Autodesk Inventor part; units mm, degrees
ref_plane "YZ Plane" through (0, 0, 0) normal (1, 0, 0) x (0, 1, 0)
ref_plane "XZ Plane" through (0, 0, 0) normal (0, 1, 0) x (-1, 0, 0)
ref_plane "XY Plane" through (0, 0, 0) normal (0, 0, 1) x (1, 0, 0)
sketch "Sketch1" plane through (0, 0, 0) normal (0, 1, 0) x (-1, 0, 0)
  circle A0 centre (0, 0) radius 3.75
  dimension "d0" = 7.5
extrude "Extrusion1" add sketch "Sketch1" along normal blind 18.4
sketch "Sketch2" plane through (0, 0, 0) normal (1, 0, 0) x (0, 1, 0)
  circle A0 centre (3.75, 0) radius 3.75
  line L0 (0, -3.75) -> (0, 3.75)
  point P0 (0, 0)
  dimension "d3" = 7.5
extrude "Extrusion2" add sketch "Sketch2" along normal blind 14.8 and the other way blind 3.75
sketch "Sketch3" plane through (0, 0, 0) normal (0, 0, 1) x (1, 0, 0)
  line L0 (17.8168, 3.75) -> (-11.5413, 3.75) construction
  line L1 (0, 19.7284) -> (0, -6.0231) construction
  line L2 (0, 3.75) -> (0, 3.75) construction
  line L3 (0, 3.75) -> (-3.75, 7.5) construction
  line L4 (-3.75, 7.5) -> (0, 3.75) construction
  line L5 (3.75, 18.4) -> (-3.75, 18.4) construction
  line L6 (0, 3.75) -> (3.75, 0) construction
  line L7 (0, 3.75) -> (0, 3.75) construction
  line L8 (3.75, 0) -> (0, 3.75) construction
  line L9 (14.8, 0) -> (14.8, 7.5) construction
  circle A0 centre (5.4, 9.15) radius 1.6
  circle A1 centre (5.4, 9.15) radius 3
  point P0 (0, 0)
  point P1 (0, 18.4)
  point P2 (14.8, 3.75)
  dimension "d8" = 5.4
  dimension "d9" = 5.4
  dimension "d10" = 3.2
  dimension "d11" = 6
extrude "Extrusion3" add sketch "Sketch3" along normal mid plane 7.4
fillet "Fillet1" radius 1 2 edges at (3.75, 18.4, 0) (14.8, 0, 0)
properties part number "Union Elbow 1-8 KQ2L01-00A SMC"
Can you work these out from the model? Positions are in its coordinate system, mm. A direction names the side the tool comes from. Give positions to 0.01 mm unless a question says otherwise; leave off trailing zeros. Loops run counter-clockwise (first coordinate to the right, second up) from the corner with the lowest first, then second, coordinate; pieces in that order, holes last. Notation, with made-up numbers: (0.5, 15.5) -> (15.5, 15.5) arc R10 ccw to (15.5, 28.5) -> close; hole circle Ø8 at (18, -8.75). An arc over 180 degrees is marked (long way). Write item = value, one per line.
1) Thinking about a two-plate mould opening in Y: for faces 4 (the cylindrical face through (7.01, 11.68, 0.05)), 5 (the flat face through (0, 0, 0)), 6 (the cylindrical face through (5.05, 7.59, 0.05)), 7 (the flat face through (7, 8, -3.7)), which applies, released by +Y, released by -Y, zero draft, split by the parting line, or undercut?
Check result:
face_4 = undercut
face_5 = released by -Y
face_6 = undercut
face_7 = zero draft
2) Suppose I cut it at B-B on z = -3. Give the number of separate pieces and of enclosed holes in the cut face, then the cut area to 3 significant figures.
Check result:
separate_pieces = 2
enclosed_holes = 1
area = 164 mm2
3) Suppose I cut it at A-A on y = 8. Write out the boundary of the cut face in (x, z).
Check result:
outline = (2.63, -3.7) -> (4.29, -3.7) -> (4.29, 3.7) -> (2.63, 3.7) -> (2.63, 2.67) arc R3.75 ccw (long way) to (2.63, -2.67) -> close; (6.51, -3.7) -> (8.17, -3.7) -> (8.17, 3.7) -> (6.51, 3.7) -> close
4) Suppose I cut it at C-C on x = 5.25. Write out the boundary of the cut face in (y, z).
Check result:
outline = (6.15, -3.7) -> (7.56, -3.7) -> (7.56, 3.7) -> (6.15, 3.7) -> (6.15, 2.88) arc R3.75 ccw (long way) to (6.15, -2.88) -> close; (10.74, -3.7) -> (12.15, -3.7) -> (12.15, 3.7) -> (10.74, 3.7) -> close
5) For faces 1 (the cylindrical face through (0.03, 1.03, 3.75)), 2 (the cylindrical face through (-2.42, 3.72, -3.75)), 3 (the cylindrical face through (-0.03, 1.03, -3.75)), which set-ups out of +Z, -Z, +X, -X, +Y, -Y let a thin tool reach every point of the face, with its end or its side?
Check result:
face_1 = +Z, -Y
face_2 = -Z, -X
face_3 = -Z, -Y
6) Will these pins go through, and if not, where does the flat tip stop? pin 1 (5 mm diameter, centred on x = 5, y = 7.5, fed in from -Z); pin 2 (1 mm diameter, centred on x = 6, y = 2, fed in from +Z); pin 3 (1.8 mm diameter, centred on x = 6.5, y = 8, fed in from +Z).
Check result:
pin_1 = -3.7
pin_2 = 3.54
pin_3 = 3.7
7) Suppose I cut it at D-D on y = 16. Write out the boundary of the cut face in (x, z), then the cut area to 3 significant figures.
Check result:
outline = circle Ø7.5 at (0, 0)
area = 44.2 mm2
8) I need wall thicknesses on L1, parallel to Y at x = 5.4, z = 1; L2, parallel to Y at x = 5.4, z = 1.25; L3, parallel to X at y = 15.5, z = 1.25. Which ranges of each line are inside material? Lowest first, please. Write a range as from..to.
Check result:
L1 = 0.14..7.55, 10.75..12.15
L2 = 0.21..7.55, 10.75..12.15
L3 = -3.54..3.54
